Can you work these out from the model? Positions are in its coordinate system, mm. Give positions to 0.01 mm unless a question says otherwise; leave off trailing zeros. Order: outer loops, then holes, each group sorted by start corner. A loop starts at its lowest first (then second) coordinate and runs counter-clockwise, first axis right, second up.
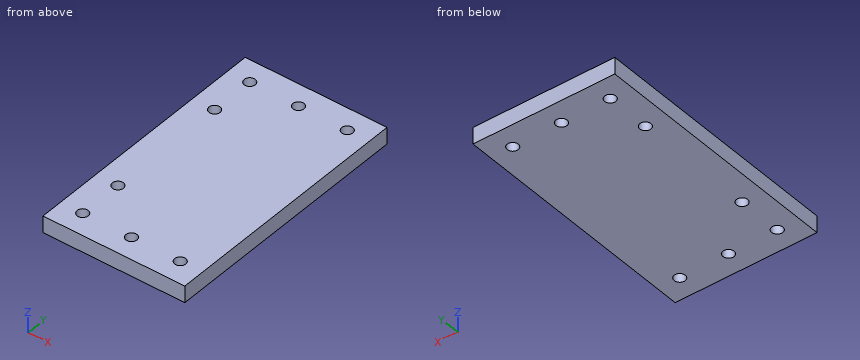
```python
from build123d import *

# Parameters (mm, degrees)
SKETCH1_W           = 64
SKETCH1_H           = 115
BOSS_EXTRUDE1_DEPTH = 3.75
SKETCH2_R           = 2.5
CUT_EXTRUDE1_DEPTH  = 67.230657554


with BuildPart() as part:
    # Sketch1 → Boss-Extrude1 (new, symmetric)
    with BuildSketch(Plane.XY):
        Rectangle(SKETCH1_W, SKETCH1_H)
    extrude(amount=BOSS_EXTRUDE1_DEPTH, both=True)

    # Sketch2 → Cut-Extrude1 (cut, symmetric)
    with BuildSketch(Plane.XY.offset(3.75)):
        with Locations((-22, 47.5)):
            Circle(SKETCH2_R)
        with Locations((0, 47.5)):
            Circle(SKETCH2_R)
        with Locations((22, 47.5)):
            Circle(SKETCH2_R)
        with Locations((-22, 27.5)):
            Circle(SKETCH2_R)
    cut_extrude1 = extrude(amount=CUT_EXTRUDE1_DEPTH, both=True, mode=Mode.SUBTRACT)

    # Mirror1: Cut-Extrude1 across plane
    add(cut_extrude1.mirror(Plane.ZX), mode=Mode.SUBTRACT)


solid = part.part
```
1) Suppose I cut it at C-C (x = 0). Please give me the cut outline in (y, z), and give its area (4 significant figures).
2) Suppose I cut it at D-D (z = -0.25). Give the number of separate pieces and of enclosed holes in the cut face, and give its area (3 significant figures).
3) Suppose I cut it at B-B (y = 27.5). Please give me the cut outline in (x, z).
4) Suppose I cut it at A-A (y = -47.5). Please give me the cut outline in (x, z), and give its area (4 significant figures).
5) If I drill on line 1 (X direction, y = -47.5, z = -1.5); line 2 (Y direction, x = 22, z = 2.5); line 3 (Y direction, x = -22, z = 0.5), over which ranges is the centre line in solid material (lowest first)?
Results:
1. outline: (-57.5, -3.75) - (-50, -3.75) - (-50, 3.75) - (-57.5, 3.75) - close; (-45, -3.75) - (45, -3.75) - (45, 3.75) - (-45, 3.75) - close; (50, -3.75) - (57.5, -3.75) - (57.5, 3.75) - (50, 3.75) - close
1. area: 787.5 mm2
2. separate pieces: 1
2. enclosed holes: 8
2. area: 7,200 mm2
3. outline: (-32, -3.75) - (-24.5, -3.75) - (-24.5, 3.75) - (-32, 3.75) - close; (-19.5, -3.75) - (32, -3.75) - (32, 3.75) - (-19.5, 3.75) - close
4. outline: (-32, -3.75) - (-24.5, -3.75) - (-24.5, 3.75) - (-32, 3.75) - close; (-19.5, -3.75) - (-2.5, -3.75) - (-2.5, 3.75) - (-19.5, 3.75) - close; (2.5, -3.75) - (19.5, -3.75) - (19.5, 3.75) - (2.5, 3.75) - close; (24.5, -3.75) - (32, -3.75) - (32, 3.75) - (24.5, 3.75) - close
4. area: 367.5 mm2
5. line 1: x = -32 to -24.5, -19.5 to -2.5, 2.5 to 19.5, 24.5 to 32
5. line 2: y = -57.5 to -50, -45 to 45, 50 to 57.5
5. line 3: y = -57.5 to -50, -45 to -30, -25 to 25, 30 to 45, 50 to 57.5
